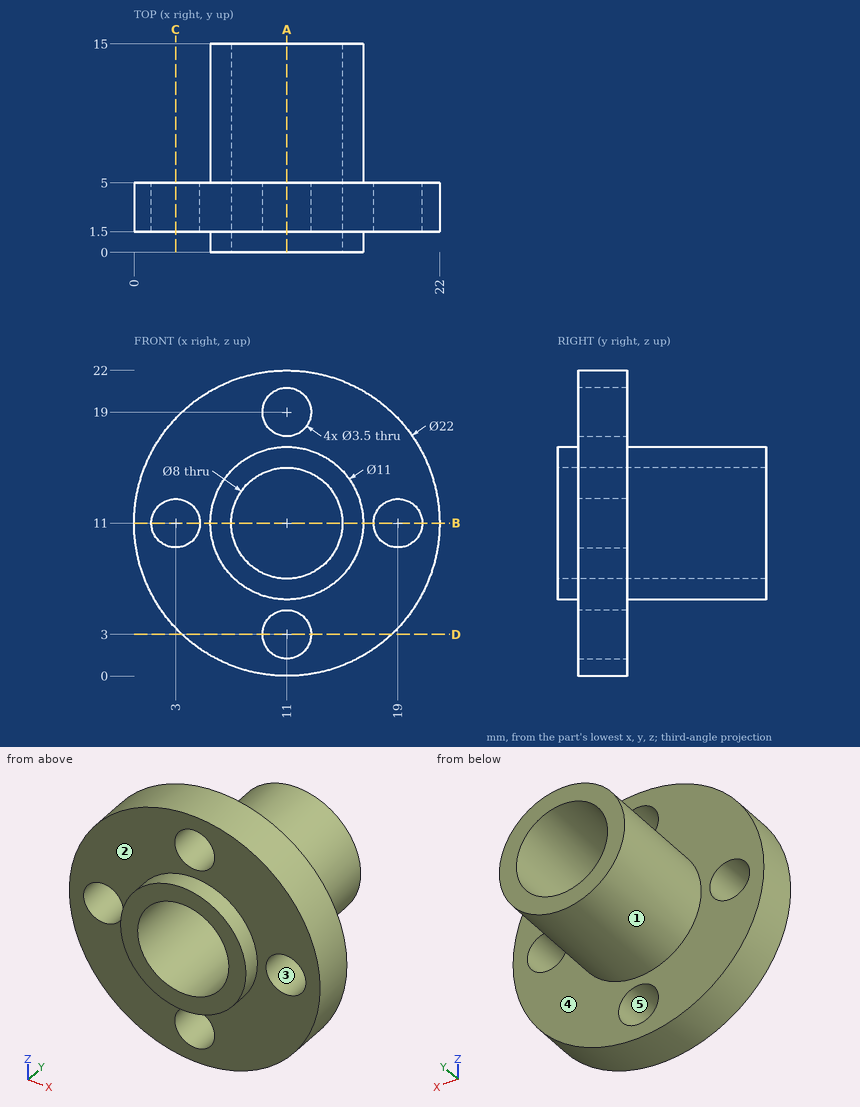
Could you check a few things on this drawing? It's one solid part, dimensions in mm from its lowest x, y, z. A direction names the side the tool comes from. Round coordinates to 2 decimals unless told otherwise and drop trailing zeros. Order: outer loops, then holes, each group sorted by start corner. A loop starts at its lowest first (then second) coordinate and runs counter-clockwise, first axis right, second up. Notation, with made-up numbers: (81.25, 64) -> (90.25, 64) arc R15 cw to (90.25, 81) -> close; hole circle Ø4 at (-31, -32.5). An arc over 180 degrees is marked (long way). One line per question, with ' | ' between items.
Q1. If we section it at C-C on x = 3: Write out the boundary of the cut face in (y, z).
Computed values:
outline: (1.5, 3.45) -> (5, 3.45) -> (5, 9.25) -> (1.5, 9.25) -> close; (1.5, 12.75) -> (5, 12.75) -> (5, 18.55) -> (1.5, 18.55) -> close
Q2. If we section it at A-A on x = 11: Write out the boundary of the cut face in (y, z), plus the area to 3 significant figures.
Computed values:
outline: (0, 5.5) -> (1.5, 5.5) -> (1.5, 4.75) -> (5, 4.75) -> (5, 5.5) -> (15, 5.5) -> (15, 7) -> (0, 7) -> close; (0, 15) -> (15, 15) -> (15, 16.5) -> (5, 16.5) -> (5, 17.25) -> (1.5, 17.25) -> (1.5, 16.5) -> (0, 16.5) -> close; (1.5, 0) -> (5, 0) -> (5, 1.25) -> (1.5, 1.25) -> close; (1.5, 20.75) -> (5, 20.75) -> (5, 22) -> (1.5, 22) -> close | area: 59.0 mm²
Q3. Which directions (+Z, -Z, +X, -X, +Y, -Y) give clear straight access to the entire face, cutting with the end or side of a thin tool? Please do the marked faces 4 and 5.
Computed values:
face 4: +Y | face 5: +Y, -Y
Q4. If we section it at B-B on z = 11: Write out the boundary of the cut face in (x, y).
Computed values:
outline: (0, 1.5) -> (1.25, 1.5) -> (1.25, 5) -> (0, 5) -> close; (4.75, 1.5) -> (5.5, 1.5) -> (5.5, 0) -> (7, 0) -> (7, 15) -> (5.5, 15) -> (5.5, 5) -> (4.75, 5) -> close; (15, 0) -> (16.5, 0) -> (16.5, 1.5) -> (17.25, 1.5) -> (17.25, 5) -> (16.5, 5) -> (16.5, 15) -> (15, 15) -> close; (20.75, 1.5) -> (22, 1.5) -> (22, 5) -> (20.75, 5) -> close
Q5. I'm going to push flat-ended pins straight in: pin 1 (1 mm diameter, centred on x = 2, z = 5.5, fed in from -Y); pin 2 (5 mm diameter, centred on y = 4.5, z = 16, fed in from -X); pin 3 (5 mm diameter, centred on x = 11, z = 11, fed in from +Y); pin 4 (8 mm diameter, centred on x = 3.5, y = 6, fed in from +Z). Where does each tip first touch, or does it pass through?
Computed values:
pin 1: y = 1.5 | pin 2: x = 0.29 | pin 3: through | pin 4: z = 21.38
Q6. We'd pull the mould along X, two halves only. Please class the marked faces 1, 2 and 3: released by +X, released by -X, zero draft, split by the parting line, or undercut.
Computed values:
face 1: split by the parting line | face 2: zero draft | face 3: undercut
Q7. If we section it at D-D on z = 3: Write out the boundary of the cut face in (x, y), plus the area to 3 significant figures.
Computed values:
outline: (3.45, 1.5) -> (9.25, 1.5) -> (9.25, 5) -> (3.45, 5) -> close; (12.75, 1.5) -> (18.55, 1.5) -> (18.55, 5) -> (12.75, 5) -> close | area: 40.6 mm²
Q8. If I drill on line 1 (X direction, y = 3.7, z = 11); line 2 (Y direction, x = 5.25, z = 2); line 3 (Z direction, x = 13, y = 6.5), over which ranges is the centre line in solid material (lowest first)? Write a range as from..to.
Computed values:
line 1: 0..1.25, 4.75..7, 15..17.25, 20.75..22 | line 2: 1.5..5 | line 3: 5.88..7.54, 14.46..16.12
